from build123d import *

# Parameters (mm, degrees)
SKETCH2_R   = 12.7
SKETCH2_R_2 = 9.525


with BuildPart() as part:
    # Sweep-Thin1: sweep along a path in Sketch1
    with BuildLine(Plane.XY) as sweep_thin1_path:
        Line((0, 0), (0, -50.8))
        ThreePointArc((0, -50.8), (81.460512212, -132.260512212), (162.921024424, -50.8))
        Line((162.921024424, -50.8), (162.921024424, 0))
    # Sketch2 → Sweep-Thin1 (sweep)
    with BuildSketch(Plane(origin=(0, 0, 0), x_dir=(1, 0, 0), z_dir=(0, 1, 0))):
        Circle(SKETCH2_R)
        Circle(SKETCH2_R_2, mode=Mode.SUBTRACT)
    sweep(path=sweep_thin1_path.line)


solid = part.part
Design review of the part built by this model. Coordinates are the model's own, in mm. A direction names the side the tool comes from. Round coordinates to 2 decimals unless told otherwise and drop trailing zeros. Order: outer loops, then holes, each group sorted by start corner. A loop starts at its lowest first (then second) coordinate and runs counter-clockwise, first axis right, second up. Notation, with made-up numbers: M 74.25,84.5 L 79.25,84.5 A22 ccw 79.25,105.5 Z; hole C 36.5,3.25 d2. An arc over 180 degrees is marked long. Answer as CSV lines item,"result". Start each with the question number.
1) For pin 1 Ø3 at (y, z) = (-118, 1.5) entering from -X; pin 2 Ø1 at (x, z) = (65.5, 6) entering from +Y; pin 3 Ø1 at (x, z) = (106.5, 2) entering from +Y, all flat-tipped, find the tip position at first contact; note any pin that passes through.
2) Tool access review of faces 4 (the face through (171.45, 0, -4.64)), 5 (the face through (170.48, -25.044, -5.796)): name each direction out of +Z, -Z, +X, -X, +Y, -Y from which nothing blocks a thin tool from reaching the whole face with its end or side.
3) The part is to be moulded in two halves that separate along Z. For faces 1 (the face through (-7.559, -25.756, -5.796)), 2 (the face through (9, 0, 5)), 3 (the face through (-2.75, -25.76, -12.4)), say which applies: +Z half, -Z half, draft (parallel to the pull), parting line (faces both ways), or undercut.
4) Wall thickness on line 1 along X through (y, z) = (-35, 0.75); line 2 along Z through (x, y) = (0, -19) (3 decimals); line 3 along X through (y, z) = (-24, -8.5): over which ranges is each line inside the solid? List them lowest first. Write a range as [from, to].
5) Add section A-A (z = 0). Give the boundary of the cut face in (x, y) (3 decimals), then the cut area to 3 significant figures.
6) Add section B-B (y = -18.5). Give the boundary of the cut face in (x, z) (3 decimals).
7) Add section C-C (y = -92.5). Give the number of separate pieces and of enclosed holes in the cut face, then the cut area to 3 significant figures.
Resolved:
1,pin 1,"x = 14.12"
1,pin 2,"y = -118.94"
1,pin 3,"y = -114.8"
2,face 4,"+Z, -Z, +X, -X, +Y"
2,face 5,"+Y"
3,face 1,"undercut"
3,face 2,"draft"
3,face 3,"parting line"
4,line 1,"[-12.68, -9.5], [9.5, 12.68], [150.24, 153.43], [172.42, 175.6]"
4,line 2,"[-12.7, -9.525], [9.525, 12.7]"
4,line 3,"[-9.44, -4.3], [4.3, 9.44], [153.48, 158.62], [167.22, 172.36]"
5,outline,"M -12.7,-50.8 A94.161 ccw 175.621,-50.8 L 175.621,0 L 172.446,0 L 172.446,-50.8 A90.986 cw -9.525,-50.8 L -9.525,0 L -12.7,0 Z; M 9.525,-50.8 A71.936 ccw 153.396,-50.8 L 153.396,0 L 150.221,0 L 150.221,-50.8 A68.761 cw 12.7,-50.8 L 12.7,0 L 9.525,0 Z"
5,area,"2,270 mm^2"
6,outline,"C 0,0 d25.4; C 162.921,0 d25.4; hole C 0,0 d19.05; hole C 162.921,0 d19.05"
7,separate pieces,"2"
7,enclosed holes,"2"
7,area,"520 mm^2"
